Geometry: final body of the model. Coordinates: model frame, mm. Coordinates: 2 decimals unless noted, no trailing zeros. Write each loop counter-clockwise with the first axis right and the second up, starting at its lowest first coordinate (ties: lowest second). Pieces come first, ordered by that corner, then holes. Notation, with made-up numbers: (-3, -7.75) -> (5, -7.75) arc R7 ccw to (5, -1.75) -> close; hole circle Ø3 at (-2, 20). An arc over 180 degrees is marked (long way). Answer as a JSON object with one key per item and string values. Group by question number.
```python
from build123d import *

# Parameters (mm, degrees)
DODANIE_WYCI_GNI_CIE1_DEPTH = 1.25


with BuildPart() as part:
    # Wyciągnięcie po ścieżce1: sweep along a path in Szkic1
    with BuildLine(Plane(origin=(0, 0, 0), x_dir=(0, 0, -1), z_dir=(1, 0, 0))) as wyci_gni_cie_po_cie_ce1_path:
        Line((0, 0), (-12, 0))
        ThreePointArc((-12, 0), (-12.485362672, -0.146955992), (-12.807692308, -0.538461538))
        ThreePointArc((-12.807692308, -0.538461538), (-14.374562589, -1.372812946), (-15.5, 0))
    # Szkic2 → Wyciągnięcie po ścieżce1 (sweep)
    with BuildSketch(Plane.XY):
        with BuildLine():
            Line((-0.7, -0.1), (0.7, -0.1))
            ThreePointArc((0.7, -0.1), (0, -0.8), (-0.7, -0.1))
        make_face()
    wyci_gni_cie_po_cie_ce1 = sweep(path=wyci_gni_cie_po_cie_ce1_path.line)

    # Lustro1: Wyciągnięcie po ścieżce1 across plane
    add(wyci_gni_cie_po_cie_ce1.mirror(Plane.ZX))

    # Szkic3 → Dodanie-wyciągnięcie1 (add)
    with BuildSketch(Plane(origin=(0, 0, 0), x_dir=(-1, 0, 0), z_dir=(0, 0, -1))):
        with BuildLine():
            Line((0.7, 0.1), (-0.7, 0.1))
            ThreePointArc((-0.7, 0.1), (0, 0.8), (0.7, 0.1))
        make_face()
    extrude(amount=DODANIE_WYCI_GNI_CIE1_DEPTH)


solid = part.part
```
Item 1: Section B-B on z = 8.75. Output: boundary loops of the cut face in (x, y).
Item 2: Contact query for a flat-ended pin moving along its axis: pin 1 (0.6 mm diameter, centred on x = 0, y = -0.5, fed in from -Z). Output: stop coordinate, or through.
Item 3: Section A-A on x = 0. Output: boundary loops of the cut face in (y, z) (3 decimals).
Item 4: Ray query, L1, parallel to Z at x = 0.15, y = -1.05; L2, parallel to Y at x = 0.4, z = 14.75; L3, parallel to Y at x = -0.35, z = 3.5. Return the intervals inside material, ascending. Write a range as [from, to].
Item 5: Mould query, pull axis Y, two halves, no side actions, for faces 1 (the cylindrical face through (0, 0.8, 5.5)), 2 (the flat face through (0, -0.1, 6)), 3 (the cylindrical face through (0, -0.8, 6.1)). Classes: +Y half, -Y half, draft (parallel to the pull), parting line (faces both ways), or undercut.
Answer sheet:
{
 "1": {"outline": "(-0.7, -0.1) arc R0.7 ccw to (0.7, -0.1) -> close; (-0.7, 0.1) -> (0.7, 0.1) arc R0.7 ccw to start"},
 "2": {"pin 1": "stops at z = 0"},
 "3": {"outline": "(-0.846, 12.069) arc R0.075 cw to (-0.8, 12) -> (-0.8, 0) -> (-0.1, 0) -> (-0.1, 12) arc R0.775 ccw to (-0.577, 12.715) arc R1.5 cw (long way) to (0.577, 12.715) arc R0.775 ccw to (0.1, 12) -> (0.1, -1.25) -> (0.8, -1.25) -> (0.8, 12) arc R0.075 cw to (0.846, 12.069) arc R2.2 ccw (long way) to start"},
 "4": {"L1": "z = [12.19, 13.03], [15.17, 16.01]", "L2": "y = [-1.97, -1.35], [1.35, 1.97]", "L3": "y = [-0.71, -0.1], [0.1, 0.71]"},
 "5": {"face 1": "+Y half", "face 2": "undercut", "face 3": "-Y half"}
}
